Build history of the part. All positions in model axes, mm. A direction names the side the tool comes from. Round coordinates to 2 decimals unless told otherwise and drop trailing zeros. Write each loop counter-clockwise with the first axis right and the second up, starting at its lowest first coordinate (ties: lowest second). Pieces come first, ordered by that corner, then holes. Notation, with made-up numbers: (-27.75, -30.5) -> (-15.75, -30.5) arc R17 cw to (-15.75, -5.5) -> close; hole circle Ø9 at (0.5, -16). An arc over 180 degrees is marked (long way). One line per question, with ' | ' between items.
from build123d import *

# Parameters (mm, degrees)
SKETCH_1_R      = 2
SKETCH_1_W      = 10
SKETCH_1_H      = 10
EXTRUDE_1_DEPTH = 3


with BuildPart() as part:
    # Эскиз1 → Бобышка-Вытянуть1 (new body)
    with BuildSketch(Plane.XY):
        with BuildLine():
            Line((13.869679809, 46.9), (26.5, 46.9))
            ThreePointArc((26.5, 46.9), (30.035533906, 45.435533906), (31.5, 41.9))
            Line((31.5, 41.9), (31.5, -41.9))
            ThreePointArc((31.5, -41.9), (30.035533906, -45.435533906), (26.5, -46.9))
            Line((26.5, -46.9), (-26.5, -46.9))
            ThreePointArc((-26.5, -46.9), (-30.035533906, -45.435533906), (-31.5, -41.9))
            Line((-31.5, -41.9), (-31.5, 41.9))
            ThreePointArc((-31.5, 41.9), (-30.035533906, 45.435533906), (-26.5, 46.9))
            Line((-26.5, 46.9), (-13.869679809, 46.9))
            ThreePointArc((-13.869679809, 46.9), (-11.041252684, 48.071572875), (-9.869679809, 50.9))
            Line((-9.869679809, 50.9), (-9.869679809, 52.9))
            ThreePointArc((-9.869679809, 52.9), (-8.698106934, 55.728427125), (-5.869679809, 56.9))
            Line((-5.869679809, 56.9), (5.869679809, 56.9))
            ThreePointArc((5.869679809, 56.9), (8.698106934, 55.728427125), (9.869679809, 52.9))
            Line((9.869679809, 52.9), (9.869679809, 50.9))
            ThreePointArc((9.869679809, 50.9), (11.041252684, 48.071572875), (13.869679809, 46.9))
        make_face()
        with Locations((-5.869679809, 51.9)):
            Circle(SKETCH_1_R, mode=Mode.SUBTRACT)
        with Locations((5.869679809, 51.9)):
            Circle(SKETCH_1_R, mode=Mode.SUBTRACT)
        with Locations((9.5, -2.5)):
            Circle(SKETCH_1_R, mode=Mode.SUBTRACT)
        with Locations((-9.5, -2.5)):
            Circle(SKETCH_1_R, mode=Mode.SUBTRACT)
        with Locations((-9.5, 7.75)):
            Circle(SKETCH_1_R, mode=Mode.SUBTRACT)
        with Locations((9.5, 7.75)):
            Circle(SKETCH_1_R, mode=Mode.SUBTRACT)
        Rectangle(SKETCH_1_W, SKETCH_1_H, mode=Mode.SUBTRACT)
    extrude(amount=EXTRUDE_1_DEPTH)


solid = part.part
(1) Slice it at B-B (z = 1.05). Write the cut outline in (x, y).
Calculated:
outline: (-31.5, -41.9) arc R5 ccw to (-26.5, -46.9) -> (26.5, -46.9) arc R5 ccw to (31.5, -41.9) -> (31.5, 41.9) arc R5 ccw to (26.5, 46.9) -> (13.87, 46.9) arc R4 cw to (9.87, 50.9) -> (9.87, 52.9) arc R4 ccw to (5.87, 56.9) -> (-5.87, 56.9) arc R4 ccw to (-9.87, 52.9) -> (-9.87, 50.9) arc R4 cw to (-13.87, 46.9) -> (-26.5, 46.9) arc R5 ccw to (-31.5, 41.9) -> close; hole circle Ø4 at (-9.5, -2.5); hole circle Ø4 at (-9.5, 7.75); hole circle Ø4 at (-5.87, 51.9); hole (-5, -5) -> (5, -5) -> (5, 5) -> (-5, 5) -> close; hole circle Ø4 at (5.87, 51.9); hole circle Ø4 at (9.5, -2.5); hole circle Ø4 at (9.5, 7.75)
(2) 3-axis set-ups, long thin cutter, end or side, ignore diameter. For faces 4 (the flat face through (20, 46.9, 1)), 5 (the flat face through (0, 6, 3)), 6 (the flat face through (31.5, 1, 1)), 7 (the flat face through (-9.87, 52, 1)), 8 (the flat face through (0, 5, 1)): which of +Z, -Z, +X, -X, +Y, -Y reach the whole face in a straight line?
Calculated:
face 4: +Z, -Z, +X, +Y | face 5: +Z, +X, -X, +Y, -Y | face 6: +Z, -Z, +X, +Y, -Y | face 7: +Z, -Z, -X, +Y | face 8: +Z, -Z
(3) Mould opens along Y. For faces 1 (the cylindrical face through (-8.729, 55.697, 1.479)), 2 (the flat face through (9.87, 52, 1)), 3 (the flat face through (0, -5, 1)) say: pulls with the +Y half, pulls with the -Y half, needs draft (parallel to the pull), parting line crosses it, or undercut.
Calculated:
face 1: pulls with the +Y half | face 2: needs draft | face 3: undercut
(4) Slice it at D-D (x = 21). Write the cut outline in (y, z).
Calculated:
outline: (-46.9, 0) -> (46.9, 0) -> (46.9, 3) -> (-46.9, 3) -> close
(5) Wall check: line 1 (Y direction, x = -2.5, z = 0.75); line 2 (Y direction, x = -9.5, z = 0.6); line 3 (Y direction, x = -22.5, z = 0.3). Give the ranges that are in metal, low to high. Write a range as from..to.
Calculated:
line 1: -46.9..-5, 5..56.9 | line 2: -46.9..-4.5, -0.5..5.75, 9.75..54.58 | line 3: -46.9..46.9
(6) Slice it at C-C (y = 51.9). Write the cut outline in (x, z).
Calculated:
outline: (-9.87, 0) -> (-7.87, 0) -> (-7.87, 3) -> (-9.87, 3) -> close; (-3.87, 0) -> (3.87, 0) -> (3.87, 3) -> (-3.87, 3) -> close; (7.87, 0) -> (9.87, 0) -> (9.87, 3) -> (7.87, 3) -> close
(7) Slice it at A-A (y = 7.75). Write the cut outline in (x, z), then the cut area to 3 significant figures.
Calculated:
outline: (-31.5, 0) -> (-11.5, 0) -> (-11.5, 3) -> (-31.5, 3) -> close; (-7.5, 0) -> (7.5, 0) -> (7.5, 3) -> (-7.5, 3) -> close; (11.5, 0) -> (31.5, 0) -> (31.5, 3) -> (11.5, 3) -> close | area: 165 mm2
(8) Drop flat-ended pins along their axis: pin 1 (0.9 mm diameter, centred on x = -19.5, z = 1, fed in from +Y); pin 2 (0.6 mm diameter, centred on y = 52.5, z = 2, fed in from -X); pin 3 (5 mm diameter, centred on x = -9.5, y = 7.75, fed in from -Z); pin 4 (1 mm diameter, centred on y = 52, z = 2, fed in from +X). Give the stop position or say it passes through.
Calculated:
pin 1: y = 46.9 | pin 2: x = -9.87 | pin 3: z = 0 | pin 4: x = 9.87
